Read the model definition and answer for the solid it produces. Units are mm, in the model's axes. Round coordinates to 2 decimals unless told otherwise and drop trailing zeros. Order: outer loops, then holes, each group sorted by start corner. A loop starts at its lowest first (then second) coordinate and runs counter-clockwise, first axis right, second up. Notation, with made-up numbers: (33, -8.5) -> (74, -8.5) arc R12 ccw to (74, 7.5) -> close; hole circle Ø7 at (-37, 25). An arc over 180 degrees is marked (long way). Answer as a JSON object with one key per item and string values. Group by question number.
Item 1: Consider probe 1 along Z at (x, y) = (220.6, 6); probe 2 along Z at (x, y) = (104, 6.5); probe 3 along Z at (x, y) = (94.1, 6.5). Determine where each line is inside the solid, lowest interval first. Write a range as from..to.
Item 2: Given P1, Ø11, axis at x = 78, z = -13, coming from the -Y side; P2, Ø9, axis at x = 197.6, z = -12.2, coming from the -Y side; P3, Ø1, axis at y = 4, z = -41, coming from the -X side, each flat-ended and moving along its own axis, determine where each tip first touches the part or whether it passes through.
Item 3: Section A-A, the plane x = 220.6 is taken. Write down the section's boundary in (y, z).
Item 4: Section D-D, the plane x = 125 is taken. Write down the section's boundary in (y, z).
Item 5: Section B-B, the plane y = 6 is taken. Count the separate pieces of the cut face and the enclosed holes in it, plus the area to 4 significant figures.
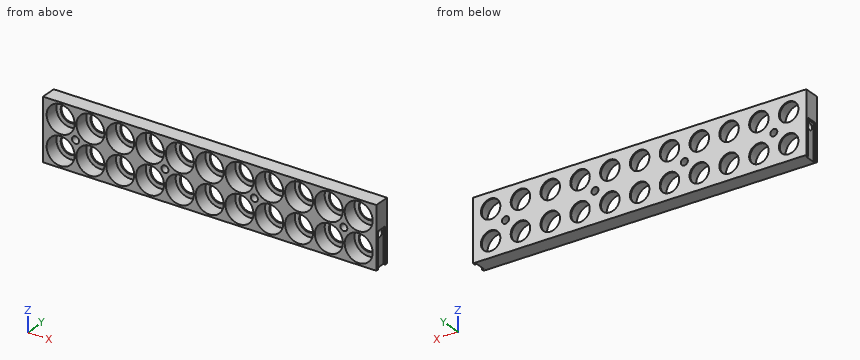
from build123d import *

# Parameters (mm, degrees)
SKETCH1_W               = 257.2
SKETCH1_H               = 47.4
BOSS_EXTRUDE1_DEPTH     = 12
CUT_EXTRUDE1_START      = -12
SKETCH2_R               = 10.8
CUT_EXTRUDE1_DEPTH      = 11
SKETCH17_R              = 7.5
CUT_EXTRUDE5_DEPTH      = 262.806417034
LPATTERN1_COUNT         = 2
LPATTERN1_PITCH         = 23
LPATTERN1_COUNT_DIR2    = 11
LPATTERN1_PITCH_DIR2    = 23
ADVANCEDHOLE1_OUTLINE_R = 2.7
ADVANCEDHOLE1_DEPTH     = 12
SKETCH9_W               = 27.7
SKETCH9_H               = 8
CUT_EXTRUDE4_DEPTH      = 1.5


# Read off the part's stored shape, not the designer's step: AdvancedHole1, AdvancedHole3
with BuildPart() as part:
    # Sketch1 → Boss-Extrude1 (new body)
    with BuildSketch(Plane(origin=(0, 0, 0), x_dir=(1, 0, 0), z_dir=(0, 1, 0))):
        with Locations((128.6, 23.7)):
            Rectangle(SKETCH1_W, SKETCH1_H)
    extrude(amount=BOSS_EXTRUDE1_DEPTH)

    # Sketch2 → Cut-Extrude1 (cut)
    with BuildSketch(Plane(origin=(0, 12, 0), x_dir=(1, 0, 0), z_dir=(0, 1, 0)).offset(CUT_EXTRUDE1_START)):
        with Locations(Location((13.6, 12.2, 0), (0, 0, 90))):
            Circle(SKETCH2_R)
    cut_extrude1 = extrude(amount=CUT_EXTRUDE1_DEPTH, mode=Mode.SUBTRACT)

    # Sketch17 → Cut-Extrude5 (cut, through all)
    with BuildSketch(Plane(origin=(0, 12, 0), x_dir=(1, 0, 0), z_dir=(0, 1, 0))):
        with Locations(Location((13.6, 12.2, 0), (0, 0, 270))):
            Circle(SKETCH17_R)
    cut_extrude5 = extrude(amount=-CUT_EXTRUDE5_DEPTH, mode=Mode.SUBTRACT)

    # LPattern1: Cut-Extrude1, Cut-Extrude5 2 × 11
    with Locations(*[(j * LPATTERN1_PITCH_DIR2, 0, -i * LPATTERN1_PITCH) for i in range(LPATTERN1_COUNT) for j in range(LPATTERN1_COUNT_DIR2) if (i, j) != (0, 0)]):
        add(cut_extrude1, mode=Mode.SUBTRACT)
        add(cut_extrude5, mode=Mode.SUBTRACT)

    # AdvancedHole1 outline → AdvancedHole1 (cut)
    with BuildSketch(Plane(origin=(0, 0, 0), x_dir=(1, 0, 0), z_dir=(0, 1, 0))):
        with Locations((163.1, 23.7)):
            Circle(ADVANCEDHOLE1_OUTLINE_R)
        with Locations((94.1, 23.7)):
            Circle(ADVANCEDHOLE1_OUTLINE_R)
        with Locations((25.1, 23.7)):
            Circle(ADVANCEDHOLE1_OUTLINE_R)
        with Locations((232.1, 23.7)):
            Circle(ADVANCEDHOLE1_OUTLINE_R)
    extrude(amount=ADVANCEDHOLE1_DEPTH, mode=Mode.SUBTRACT)

    # Sketch9 → Cut-Extrude4 (cut)
    with BuildSketch(Plane.ZY):
        with Locations((-33.55, 6)):
            Rectangle(SKETCH9_W, SKETCH9_H)
    cut_extrude4 = extrude(amount=-CUT_EXTRUDE4_DEPTH, mode=Mode.SUBTRACT)

    # AdvancedHole3 outline → AdvancedHole3 (revolve, cut)
    with BuildSketch(Plane(origin=(0, 6, -23.7), x_dir=(0, 1, 0), z_dir=(0, 0, -1))):
        Polygon((2.615, 1.5), (2.524951623, 5.39), (0, 5.39), (0, 1.5), align=None)
    advancedhole3 = revolve(axis=Axis((0, 6, -23.7), (1, 0, 0)), mode=Mode.SUBTRACT)

    # Mirror1: Cut-Extrude4, AdvancedHole3 across plane
    add(cut_extrude4.mirror(Plane(origin=(128.6, 0, 0), x_dir=(0, 0, 1), z_dir=(1, 0, 0))), mode=Mode.SUBTRACT)
    add(advancedhole3.mirror(Plane(origin=(128.6, 0, 0), x_dir=(0, 0, 1), z_dir=(1, 0, 0))), mode=Mode.SUBTRACT)


solid = part.part
Values found:
{
 "1": {"probe 1": "-47.4..-46, -24.4..-23, -1.4..0", "probe 2": "-47.4..-45.88, -24.52..-22.88, -1.52..0", "probe 3": "-47.4..-26.4, -21..0"},
 "2": {"P1": "y = 11", "P2": "through", "P3": "x = 1.5"},
 "3": {"outline": "(0, -47.4) -> (12, -47.4) -> (12, -42.7) -> (11, -42.7) -> (11, -46) -> (0, -46) -> close; (0, -24.4) -> (11, -24.4) -> (11, -27.7) -> (12, -27.7) -> (12, -19.7) -> (11, -19.7) -> (11, -23) -> (0, -23) -> close; (0, -1.4) -> (11, -1.4) -> (11, -4.7) -> (12, -4.7) -> (12, 0) -> (0, 0) -> close"},
 "4": {"outline": "(0, -47.4) -> (12, -47.4) -> (12, -41.78) -> (11, -41.78) -> (11, -45.38) -> (0, -45.38) -> close; (0, -25.02) -> (11, -25.02) -> (11, -28.62) -> (12, -28.62) -> (12, -18.78) -> (11, -18.78) -> (11, -22.38) -> (0, -22.38) -> close; (0, -2.02) -> (11, -2.02) -> (11, -5.62) -> (12, -5.62) -> (12, 0) -> (0, 0) -> close"},
 "5": {"separate pieces": "1", "enclosed holes": "26", "area": "3,915 mm2"}
}
